Check sheet for the modelled part. Datum: model origin and axes. Units: mm. Face numbers are marked on the shaded views. Give positions to 0.01 mm unless a question says otherwise; leave off trailing zeros. Write each loop counter-clockwise with the first axis right and the second up, starting at its lowest first coordinate (ties: lowest second). Pieces come first, ordered by that corner, then holes. Notation, with made-up numbers: M 39,35.25 L 81,35.25 A29 ccw 81,72.25 Z; hole C -12.5,88.5 d9. An arc over 180 degrees is marked long. Write item = value, one per line. Start each with the question number.
1) Sectioned sample at B-B, the plane x = 39. Record the cut outline in (y, z), then the cut area to 3 significant figures.
2) Scan lines: L1, parallel to Y at x = -111, z = 202.5; L2, parallel to Y at x = 129.5, z = 203; L3, parallel to Y at x = -84, z = 230.5. Record each from-to range of solid material in increasing order.
3) Draft check along X on the marked faces 1, 2, 3 and 4. Enter one of: pulls with the +X half, pulls with the -X half, needs draft (parallel to the pull), parting line crosses it, or undercut.
4) Gauge pin test, flat ends, axial feed: pin 1 (10 mm diameter, centred on x = 212.5, y = 230, fed in from +Z); pin 2 (15 mm diameter, centred on x = 108, y = 9, fed in from +Z); pin 3 (1 mm diameter, centred on x = -227.5, y = -63, fed in from +Z). Record the tip position at first contact, or that the pin passes through.
5) Sectioned sample at D-D, the plane z = 340.5. Record the cut outline in (x, y), then the cut area to 3 significant figures.
6) Sectioned sample at A-A, the plane z = 131. Count the separate pieces of the cut face and the enclosed holes in it, then the cut area to 3 significant figures.
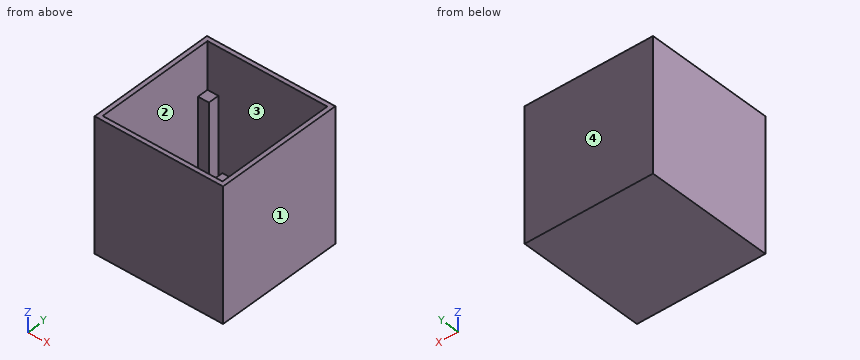
from build123d import *

# Parameters (mm, degrees)
F1_DEPTH = 20
F0_W     = 600
F0_H     = 600
F2_DEPTH = 620
F0_W_2   = 50.8
F0_H_2   = 101.6
F0_W_3   = 101.6
F0_H_3   = 50.8
F3_DEPTH = 220
F0_H_4   = 203.2
F0_W_4   = 203.2
F4_DEPTH = 70.8
F5_DEPTH = 400


with BuildPart() as f1:
    # F0 (on Top) → F1 (new body)
    with BuildSketch(Plane.XY):
        Polygon((26, 280), (-229.2, 280), (-229.2, 229.2), (-229.2, 26), (-280, 26), (-280, -229.2), (-229.2, -229.2), (-26, -229.2), (-26, -280), (229.2, -280), (229.2, -229.2), (229.2, -26), (280, -26), (280, 229.2), (229.2, 229.2), (26, 229.2), align=None)
        Polygon((-130.8, 130.8), (-80, 130.8), (21.6, 130.8), (130.8, 130.8), (130.8, 80), (130.8, -21.6), (130.8, -130.8), (80, -130.8), (-21.6, -130.8), (-130.8, -130.8), (-130.8, -80), (-130.8, 21.6), align=None, mode=Mode.SUBTRACT)
        Polygon((21.6, 80), (-80, 80), (-80, 130.8), (-130.8, 130.8), (-130.8, 21.6), (-80, 21.6), (-80, -80), (-130.8, -80), (-130.8, -130.8), (-21.6, -130.8), (-21.6, -80), (80, -80), (80, -130.8), (130.8, -130.8), (130.8, -21.6), (80, -21.6), (80, 80), (130.8, 80), (130.8, 130.8), (21.6, 130.8), align=None)
    extrude(amount=F1_DEPTH)

    # F0 (on Top) → F2 (join)
    with BuildSketch(Plane.XY):
        Rectangle(F0_W, F0_H)
        Polygon((-280, 229.2), (-280, 280), (-229.2, 280), (26, 280), (229.2, 280), (280, 280), (280, 229.2), (280, -26), (280, -229.2), (280, -280), (229.2, -280), (-26, -280), (-229.2, -280), (-280, -280), (-280, -229.2), (-280, 26), align=None, mode=Mode.SUBTRACT)
    extrude(amount=F2_DEPTH)

    # F0 (on Top) → F3 (join)
    with BuildSketch(Plane.XY):
        with Locations((-105.4, -29.2)):
            Rectangle(F0_W_2, F0_H_2)
        with Locations((-29.2, 105.4)):
            Rectangle(F0_W_3, F0_H_3)
        with Locations((105.4, 29.2)):
            Rectangle(F0_W_2, F0_H_2)
        with Locations((29.2, -105.4)):
            Rectangle(F0_W_3, F0_H_3)
    extrude(amount=F3_DEPTH)

    # F0 (on Top) → F4 (join)
    with BuildSketch(Plane.XY):
        with Locations((-254.6, 127.6)):
            Rectangle(F0_W_2, F0_H_4)
        with Locations((254.6, -127.6)):
            Rectangle(F0_W_2, F0_H_4)
        with Locations((-127.6, -254.6)):
            Rectangle(F0_W_4, F0_H_3)
        with Locations((127.6, 254.6)):
            Rectangle(F0_W_4, F0_H_3)
    extrude(amount=F4_DEPTH)

    # F0 (on Top) → F5 (join)
    with BuildSketch(Plane.XY):
        with Locations((-254.6, 254.6)):
            Rectangle(F0_W_2, F0_H_3)
        with Locations((-254.6, -254.6)):
            Rectangle(F0_W_2, F0_H_3)
        with Locations((254.6, -254.6)):
            Rectangle(F0_W_2, F0_H_3)
        with Locations((254.6, 254.6)):
            Rectangle(F0_W_2, F0_H_3)
    extrude(amount=F5_DEPTH)


solid = f1.part
Data:
q1.outline = M -300,0 L 300,0 L 300,620 L 280,620 L 280,70.8 L 229.2,70.8 L 229.2,20 L -80,20 L -80,220 L -130.8,220 L -130.8,20 L -280,20 L -280,620 L -300,620 Z
q1.area = 48,700 mm2
q2.L1 = -300 to -280, -80 to 21.6, 280 to 300
q2.L2 = -300 to -280, -21.6 to 80, 280 to 300
q2.L3 = -300 to -280, 280 to 300
q3.face_1 = pulls with the +X half
q3.face_2 = undercut
q3.face_3 = undercut
q3.face_4 = needs draft
q4.pin_1 = 70.8
q4.pin_2 = 220
q4.pin_3 = 20
q5.outline = M -300,-300 L 300,-300 L 300,300 L -300,300 Z; hole M -280,-229.2 L -229.2,-229.2 L -229.2,-280 L 229.2,-280 L 229.2,-229.2 L 280,-229.2 L 280,229.2 L 229.2,229.2 L 229.2,280 L -229.2,280 L -229.2,229.2 L -280,229.2 Z
q5.area = 56,700 mm2
q6.separate_pieces = 5
q6.enclosed_holes = 1
q6.area = 77,400 mm2
